Job drawing, mm, ordinate dimensions from the low corner. One solid piece. Give positions to 0.01 mm unless a question says otherwise; leave off trailing zeros. Loops run counter-clockwise (first coordinate to the right, second up) from the corner with the lowest first, then second, coordinate; pieces in that order, holes last.
Item 1: Saw through at A-A on x = 25.4. Give the cut face in (y, z), plus the area to 3 significant figures.
Item 2: Drop flat-ended pins along their axis: P1, Ø10.5, axis at x = 260.35, y = 117.4, coming from the -Z side; P2, Ø6, axis at x = 25.4, y = 117.4, coming from the +Z side. Give the stop position or say it passes through.
Item 3: Probe probe 1 along Y at (x, z) = (260.35, 4.75); probe 2 along X at (y, z) = (104.5, 4.75). List the from-to ranges inside material, lowest first.
Item 4: Saw through at B-B on y = 92. Give the cut face in (x, z).
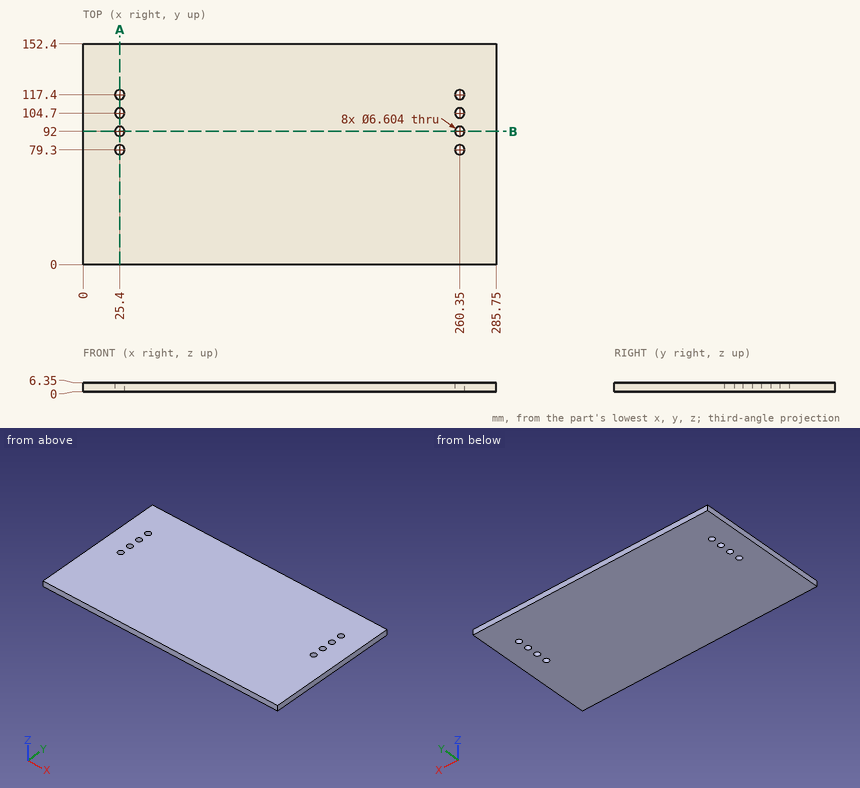
Results below:
1. outline: (0, 0) - (76, 0) - (76, 6.35) - (0, 6.35) - close; (82.6, 0) - (88.7, 0) - (88.7, 6.35) - (82.6, 6.35) - close; (95.3, 0) - (101.4, 0) - (101.4, 6.35) - (95.3, 6.35) - close; (108, 0) - (114.1, 0) - (114.1, 6.35) - (108, 6.35) - close; (120.7, 0) - (152.4, 0) - (152.4, 6.35) - (120.7, 6.35) - close
1. area: 800 mm2
2. P1: stops at z = 0
2. P2: passes through
3. probe 1: y = 0 to 76, 82.6 to 88.7, 95.3 to 101.4, 108 to 114.1, 120.7 to 152.4
3. probe 2: x = 0 to 22.1, 28.7 to 257.05, 263.65 to 285.75
4. outline: (0, 0) - (22.1, 0) - (22.1, 6.35) - (0, 6.35) - close; (28.7, 0) - (257.05, 0) - (257.05, 6.35) - (28.7, 6.35) - close; (263.65, 0) - (285.75, 0) - (285.75, 6.35) - (263.65, 6.35) - close
